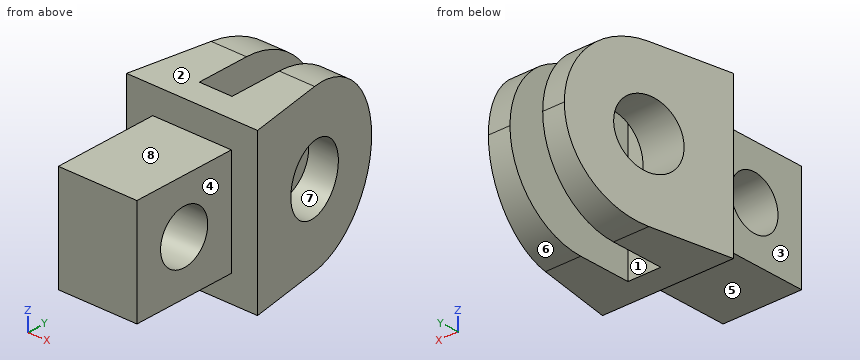
```python
from build123d import *

# Parameters (mm, degrees)
SKETCH1_W           = 80
SKETCH1_H           = 60
BOSS_EXTRUDE1_DEPTH = 40
BOSS_EXTRUDE2_DEPTH = 60
SKETCH2_R           = 25
CUT_EXTRUDE2_DEPTH  = 60
FILLET1_R           = 60
SKETCH3_R           = 20
CUT_EXTRUDE3_DEPTH  = 60


with BuildPart() as part:
    # Sketch1 → Boss-Extrude1 (new, symmetric)
    with BuildSketch(Plane(origin=(0, 0, 0), x_dir=(0, 1, 0), z_dir=(0, 0, 1))):
        with Locations((-60, 0)):
            Rectangle(SKETCH1_W, SKETCH1_H)
    extrude(amount=BOSS_EXTRUDE1_DEPTH, both=True)

    # Sketch1<3> → Boss-Extrude2 (add, symmetric)
    with BuildSketch(Plane(origin=(0, 0, 0), x_dir=(0, 1, 0), z_dir=(0, 0, 1))):
        Polygon((100, -29), (-20, -50), (-20, 50), (100, 29), (100, 12.5), (0, 12.5), (0, -12.5), (100, -12.5), align=None)
    extrude(amount=BOSS_EXTRUDE2_DEPTH, both=True)

    # Sketch2 → Cut-Extrude2 (cut, symmetric)
    with BuildSketch(Plane.YZ):
        with Locations((40, 0)):
            Circle(SKETCH2_R)
    extrude(amount=CUT_EXTRUDE2_DEPTH, both=True, mode=Mode.SUBTRACT)

    # Fillet1
    fillet1_edges = [part.edges().sort_by_distance(p)[0] for p in [
        (-20.75, 100, -60),
        (20.75, 100, -60),
        (-20.75, 100, 60),
        (20.75, 100, 60),
    ]]
    fillet(fillet1_edges, radius=FILLET1_R - 0.0001)  # a hair under: the kernel refuses the full size

    # Sketch3 → Cut-Extrude3 (cut, symmetric)
    with BuildSketch(Plane.YZ.offset(30)):
        with Locations((-60, 0)):
            Circle(SKETCH3_R)
    extrude(amount=CUT_EXTRUDE3_DEPTH, both=True, mode=Mode.SUBTRACT)


solid = part.part
```
Design review of the part built by this model. Coordinates are the model's own, in mm. Face numbers are marked on the shaded views. A direction names the side the tool comes from. Coordinates: 2 decimals unless noted, no trailing zeros. Write each loop counter-clockwise with the first axis right and the second up, starting at its lowest first coordinate (ties: lowest second). Pieces come first, ordered by that corner, then holes. Notation, with made-up numbers: M 86,8.5 L 119,8.5 A13 cw 119,24.5 Z; hole C 56,73.25 d10. An arc over 180 degrees is marked long. Answer as a JSON object with one key per item and string values.
Item 1: Add section B-B, the plane x = 21. State how many separate pieces and enclosed holes the cut face has, and give its area (3 significant figures).
Outcome:
{"separate pieces": "1", "enclosed holes": "2", "area": "16,000 mm²"}
Item 2: Add section C-C, the plane z = -3. Give the boundary of the cut face in (x, y).
Outcome:
{"outline": "M -50,-20 L -30,-20 L -30,-40.23 L 30,-40.23 L 30,-20 L 50,-20 L 43.84,15.18 L 12.5,15.18 L 12.5,0 L -12.5,0 L -12.5,15.18 L -43.84,15.18 Z; M -35.16,64.82 L -12.5,64.82 L -12.5,99.92 L -29.01,99.92 Z; M -30,-100 L 30,-100 L 30,-79.77 L -30,-79.77 Z; M 12.5,64.82 L 35.16,64.82 L 29.01,99.92 L 12.5,99.92 Z"}
Item 3: Insertion check: pin 1 Ø24 at (y, z) = (-76.5, -9) entering from +X; pin 2 Ø20 at (x, z) = (-0.5, -24) entering from +Y; pin 3 Ø2 at (x, y) = (1, -75.5) entering from -Z. Each pin has a flat end and moves straight along its axis. Give the tip position at first contact, or say it passes through.
Outcome:
{"pin 1": "x = 30", "pin 2": "y = 0", "pin 3": "z = -40"}
Item 4: Machinability: for the marked faces 1, 2, 3, 4 and 5, which of the approach directions +Z, -Z, +X, -X, +Y, -Y give a long, thin tool a straight path to every point of the face, cutting with its end or side? Answer none if there is none.
Outcome:
{"face 1": "+Z, -Z, +Y", "face 2": "+Z, +X, -X, +Y, -Y", "face 3": "+Z, -Z, -X, -Y", "face 4": "+Z, -Z, +X, -Y", "face 5": "-Z, +X, -X, -Y"}
Item 5: Wall thickness on probe 1 along Z at (x, y) = (30, 40); probe 2 along Z at (x, y) = (-8, -60); probe 3 along X at (y, z) = (5.5, 46): over which ranges is each line inside the solid? List them lowest first.
Outcome:
{"probe 1": "-60 to -25, 25 to 60", "probe 2": "-40 to -20, 20 to 40", "probe 3": "-45.54 to -12.5, 12.5 to 45.54"}
Item 6: Add section A-A, the plane y = -60. Give the boundary of the cut face in (x, z), and give its area (3 significant figures).
Outcome:
{"outline": "M -30,-40 L 30,-40 L 30,-20 L -30,-20 Z; M -30,20 L 30,20 L 30,40 L -30,40 Z", "area": "2,400 mm²"}
Item 7: Add section D-D, the plane y = 17.5. Give the boundary of the cut face in (x, z), and give its area (3 significant figures).
Outcome:
{"outline": "M -43.44,-60 L -12.5,-60 L -12.5,-10.9 L -43.44,-10.9 Z; M -43.44,10.9 L -12.5,10.9 L -12.5,60 L -43.44,60 Z; M 12.5,-60 L 43.44,-60 L 43.44,-10.9 L 12.5,-10.9 Z; M 12.5,10.9 L 43.44,10.9 L 43.44,60 L 12.5,60 Z", "area": "6,080 mm²"}
Item 8: Draft analysis for pull direction Z (two halves, no side actions). For the marked faces 6, 7 and 8, state which applies: pulls with the +Z half, pulls with the -Z half, needs draft (parallel to the pull), parting line crosses it, or undercut.
Outcome:
{"face 6": "pulls with the -Z half", "face 7": "undercut", "face 8": "pulls with the +Z half"}
